from build123d import *

# Parameters (mm, degrees)
F1_DEPTH = 127
F2_W     = 6.35
F2_H     = 71.12
F3_DEPTH = 69.85


with BuildPart() as f1:
    # F0 (on Front) → F1 (new body)
    with BuildSketch(Plane.XZ):
        Polygon((-43.496815, 38.881797), (-51.751815, 38.881797), (-51.751815, -40.493203), (27.623185, -40.493203), (27.623185, -32.238203), (-43.496815, -32.238203), align=None)
    extrude(amount=F1_DEPTH)

    # F2 (on face) → F3 (join)
    with BuildSketch(Plane.YZ.offset(-43.496815)):
        with Locations((-120.65, 3.321797)):
            Rectangle(F2_W, F2_H)
        with Locations((-6.35, 3.321797)):
            Rectangle(F2_W, F2_H)
    extrude(amount=F3_DEPTH)


solid = f1.part
Read the model definition and answer for the solid it produces. Units are mm, in the model's axes. A direction names the side the tool comes from. Give positions to 0.01 mm unless a question says otherwise; leave off trailing zeros. Loops run counter-clockwise (first coordinate to the right, second up) from the corner with the lowest first, then second, coordinate; pieces in that order, holes last. Notation, with made-up numbers: (14.5, 3.25) -> (42.5, 3.25) arc R17 cw to (42.5, 11.25) -> close; hole circle Ø11 at (30.25, -17.75). An arc over 180 degrees is marked (long way). Use a Markdown table: item, result.
Q1. Determine the mould class of faces 5 (the face through (-30, 0, -33)), 6 (the face through (-13, -63, -40.493)), 7 (the face through (-9, -117.475, 3)), 8 (the face through (-7, -63, -32.238)) for opening direction Y: pulls with the +Y half, pulls with the -Y half, needs draft (parallel to the pull), parting line crosses it, or undercut.
Solved:
| item | result |
|---|---|
| face 5 | pulls with the +Y half |
| face 6 | needs draft |
| face 7 | undercut |
| face 8 | undercut |
Q2. Section C-C, the plane y = -105 is taken. Determine the outline of the cut face in (x, z), then the cut area to 3 significant figures.
Solved:
| item | result |
|---|---|
| outline | (-51.75, -40.49) -> (27.62, -40.49) -> (27.62, -32.24) -> (-43.5, -32.24) -> (-43.5, 38.88) -> (-51.75, 38.88) -> close |
| area | 1,240 mm^2 |
Q3. Each of these flat-tipped pins is pushed along its axis until it touches: pin 1 (21.5 mm diameter, centred on x = -7, y = -45, fed in from +Z); pin 2 (12 mm diameter, centred on x = -36, z = -16.5, fed in from -Y) (3 decimals); pin 3 (1.6 mm diameter, centred on y = -124.5, z = 21, fed in from +X). Where does it stop, or does it pass through?
Solved:
| item | result |
|---|---|
| pin 1 | stops at z = -32.24 |
| pin 2 | stops at y = -123.825 |
| pin 3 | stops at x = 26.35 |
Q4. Section B-B, the plane z = -10 is taken. Determine the outline of the cut face in (x, y) (3 decimals).
Solved:
| item | result |
|---|---|
| outline | (-51.752, -127) -> (-43.497, -127) -> (-43.497, -123.825) -> (26.353, -123.825) -> (26.353, -117.475) -> (-43.497, -117.475) -> (-43.497, -9.525) -> (26.353, -9.525) -> (26.353, -3.175) -> (-43.497, -3.175) -> (-43.497, 0) -> (-51.752, 0) -> close |
Q5. Find the intervals of material crossed by line 1 along Y through (x, z) = (-32.5, 23) (3 decimals); line 2 along X through (y, z) = (-10.5, 29); line 3 along Z through (x, y) = (-36.5, -14), in increasing order.
Solved:
| item | result |
|---|---|
| line 1 | y = -123.825 to -117.475, -9.525 to -3.175 |
| line 2 | x = -51.75 to -43.5 |
| line 3 | z = -40.49 to -32.24 |
Q6. A tool of negligible diameter and unlimited length cuts with its end or side. For faces 1 (the face through (26.353, -121, 4)), 2 (the face through (-9, -123.825, 3)), 3 (the face through (-43.497, -2, 3)), 4 (the face through (-43.497, -63, 3)), from which of +Z, -Z, +X, -X, +Y, -Y can it reach the whole face along a straight path? Write none if from no direction.
Solved:
| item | result |
|---|---|
| face 1 | +Z, +X, +Y, -Y |
| face 2 | +Z, +X, -Y |
| face 3 | +Z, +X, +Y |
| face 4 | +Z, +X |
Q7. Section A-A, the plane x = -38 is taken. Determine the outline of the cut face in (y, z) (3 decimals).
Solved:
| item | result |
|---|---|
| outline | (-127, -40.493) -> (0, -40.493) -> (0, -32.238) -> (-3.175, -32.238) -> (-3.175, 38.882) -> (-9.525, 38.882) -> (-9.525, -32.238) -> (-117.475, -32.238) -> (-117.475, 38.882) -> (-123.825, 38.882) -> (-123.825, -32.238) -> (-127, -32.238) -> close |
